```python
from build123d import *

# Parameters (mm, degrees)
EXTRUDE_1_DEPTH     = 20
SKETCH_3_R          = 1.1
CUT_EXTRUDE_1_DEPTH = 20
CHAMFER_1_SIZE      = 1


with BuildPart() as part:
    # 草图2 → 凸台-拉伸1 (new body)
    with BuildSketch(Plane(origin=(0, 0, 0), x_dir=(1, 0, 0), z_dir=(0, 1, 0))):
        with BuildLine():
            Line((6.581223291, -1.5), (-6.581223291, -1.5))
            ThreePointArc((-6.581223291, -1.5), (-5.826905037, -3.40729771), (-4.534589287, -5))
            Line((-4.534589287, -5), (4.534589287, -5))
            ThreePointArc((4.534589287, -5), (5.826905037, -3.40729771), (6.581223291, -1.5))
        make_face()
    extrude(amount=EXTRUDE_1_DEPTH)

    # 草图3 → 切除-拉伸1 (cut)
    with BuildSketch(Plane.XY.offset(5)):
        with Locations((0, 15)):
            Circle(SKETCH_3_R)
        with Locations((0, 8)):
            Circle(SKETCH_3_R)
    extrude(amount=-CUT_EXTRUDE_1_DEPTH, mode=Mode.SUBTRACT)

    # 倒角1
    chamfer_1_edges = [part.edges().sort_by_distance(p)[0] for p in [
        (0, 0, 5),
    ]]
    chamfer(chamfer_1_edges, length=CHAMFER_1_SIZE)


solid = part.part
```
The listing builds one solid part. Answer for the finished solid, in the listing's coordinates (mm). Coordinates: 2 decimals unless noted, no trailing zeros. Loops run counter-clockwise (first coordinate to the right, second up) from the corner with the lowest first, then second, coordinate; pieces in that order, holes last. Notation, with made-up numbers: (87.5, 80) - (122.5, 80) arc R30 cw to (122.5, 117) - close; hole circle Ø2 at (72.25, -22.75). An arc over 180 degrees is marked (long way). Use a Markdown table: item, result. Add a question column.
1) Find the intervals of material crossed by line 1 (Y direction, x = 0, z = 4.35); line 2 (Y direction, x = -0.25, z = 4.8); line 3 (X direction, y = 15.75, z = 4.35), in increasing order.
2) The part is cut by section B-B, the plane x = 0. Give the vertices of the cut face in (y, z).
3) The part is cut by section C-C, the plane z = 2.2. Give the vertices of the cut face in (x, y), and give its area (3 significant figures).
4) The part is cut by section D-D, the plane y = 8.75. Give the vertices of the cut face in (x, z), and give its area (3 significant figures).
5) The mould has two halves that part along Y. Classify faces 1 (the flat face through (0, 20, 3)), 2 (the cylindrical face through (5.812, 9.86, 3.432)), 3 (the cylindrical face through (-0.238, 6.926, 3.274)), 4 (the cylindrical face through (-0.238, 13.926, 3.274)): released by +Y, released by -Y, zero draft, split by the parting line, or undercut.
6) The part is cut by section A-A, the plane y = 15. Give the vertices of the cut face in (x, z), and give its area (3 significant figures).
Here are the results:
| question | item | result |
|---|---|---|
| 1 | line 1 | y = 0.35 to 6.9, 9.1 to 13.9, 16.1 to 20 |
| 1 | line 2 | y = 0.8 to 6.93, 9.07 to 13.93, 16.07 to 20 |
| 1 | line 3 | x = -5.16 to -0.8, 0.8 to 5.16 |
| 2 | outline | (0, 1.5) - (6.9, 1.5) - (6.9, 5) - (1, 5) - (0, 4) - close; (9.1, 1.5) - (13.9, 1.5) - (13.9, 5) - (9.1, 5) - close; (16.1, 1.5) - (20, 1.5) - (20, 5) - (16.1, 5) - close |
| 3 | outline | (-6.38, 0) - (6.38, 0) - (6.38, 20) - (-6.38, 20) - close; hole circle Ø2.2 at (0, 8); hole circle Ø2.2 at (0, 15) |
| 3 | area | 248 mm^2 |
| 4 | outline | (-6.58, 1.5) - (-0.8, 1.5) - (-0.8, 5) - (-4.53, 5) arc R6.75 ccw to start; (0.8, 1.5) - (6.58, 1.5) arc R6.75 ccw to (4.53, 5) - (0.8, 5) - close |
| 4 | area | 35.0 mm^2 |
| 5 | face 1 | released by +Y |
| 5 | face 2 | zero draft |
| 5 | face 3 | undercut |
| 5 | face 4 | undercut |
| 6 | outline | (-6.58, 1.5) - (-1.1, 1.5) - (-1.1, 5) - (-4.53, 5) arc R6.75 ccw to start; (1.1, 1.5) - (6.58, 1.5) arc R6.75 ccw to (4.53, 5) - (1.1, 5) - close |
| 6 | area | 32.9 mm^2 |
